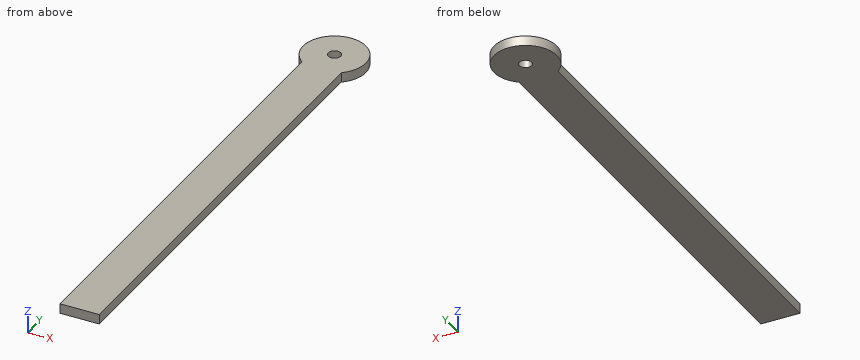
```python
from build123d import *

# Parameters (mm, degrees)
SKETCH1_W           = 12.7
SKETCH1_H           = 165.1
BOSS_EXTRUDE1_DEPTH = 3.175
SKETCH3_R           = 10.16
BOSS_EXTRUDE2_DEPTH = 3.175
SKETCH4_R           = 2.032
CUT_EXTRUDE2_DEPTH  = 168.977605129


with BuildPart() as part:
    # Sketch1 → Boss-Extrude1 (new body)
    with BuildSketch(Plane.XY):
        with Locations((0, 82.55)):
            Rectangle(SKETCH1_W, SKETCH1_H)
    extrude(amount=BOSS_EXTRUDE1_DEPTH)

    # Sketch3 → Boss-Extrude2 (add)
    with BuildSketch(Plane.XY.offset(3.175)):
        with Locations((0, 157.48)):
            Circle(SKETCH3_R)
    extrude(amount=-BOSS_EXTRUDE2_DEPTH)

    # Sketch4 → Cut-Extrude2 (cut, through all)
    with BuildSketch(Plane.XY.offset(3.175)):
        with Locations((0, 157.48)):
            Circle(SKETCH4_R)
    extrude(amount=-CUT_EXTRUDE2_DEPTH, mode=Mode.SUBTRACT)


solid = part.part
```
Here's how the part is built. I have some questions about the finished solid (model axes, mm). Coordinates: 2 decimals unless noted, no trailing zeros. Write each loop counter-clockwise with the first axis right and the second up, starting at its lowest first coordinate (ties: lowest second). Pieces come first, ordered by that corner, then holes. Notation, with made-up numbers: M 72.5,65.5 L 100.5,65.5 A23 ccw 100.5,104.5 Z; hole C -14,62.25 d7. An arc over 180 degrees is marked long. Answer as CSV lines item,"result". Start each with the question number.
Q1. Suppose I cut it at A-A, the plane y = 157.48. List the corners of the cut face in (x, z) for me (3 decimals).
Q2. Will these pins go through, and if not, where does the flat tip stop? pin 1 Ø1 at (y, z) = (70.5, 0.5) entering from +X; pin 2 Ø1.5 at (x, z) = (2, 1.5) entering from +Y.
Q3. Suppose I cut it at C-C, the plane x = 0. List the corners of the cut face in (y, z) for me (3 decimals).
Q4. Suppose I cut it at B-B, the plane z = 0.7. List the corners of the cut face in (x, y) for me, then the cut area to 3 significant figures.
Q5. I need wall thicknesses on probe 1 along Y at (x, z) = (0, 1.9); probe 2 along X at (y, z) = (157.48, 1.25); probe 3 along X at (y, z) = (139.5, 2.5). Which ranges of each line are inside material? Lowest first, please. Write a range as [from, to].
Entries:
1,outline,"M -10.16,0 L -2.032,0 L -2.032,3.175 L -10.16,3.175 Z; M 2.032,0 L 10.16,0 L 10.16,3.175 L 2.032,3.175 Z"
2,pin 1,"stops at x = 6.35"
2,pin 2,"stops at y = 167.56"
3,outline,"M 0,0 L 155.448,0 L 155.448,3.175 L 0,3.175 Z; M 159.512,0 L 167.64,0 L 167.64,3.175 L 159.512,3.175 Z"
4,outline,"M -6.35,0 L 6.35,0 L 6.35,149.55 A10.16 ccw long -6.35,149.55 Z; hole C 0,157.48 d4.06"
4,area,"2,190 mm²"
5,probe 1,"y = [0, 155.45], [159.51, 167.64]"
5,probe 2,"x = [-10.16, -2.03], [2.03, 10.16]"
5,probe 3,"x = [-6.35, 6.35]"
